Can you work these out from the model? Positions are in its coordinate system, mm. A direction names the side the tool comes from. Round coordinates to 2 decimals unless told otherwise and drop trailing zeros. Loops run counter-clockwise (first coordinate to the right, second up) from the corner with the lowest first, then second, coordinate; pieces in that order, holes last. Notation, with made-up numbers: M 2.25,49 L 13.25,49 A25 cw 13.25,70 Z; hole C 6.25,16 d6. An arc over 180 degrees is marked long. Answer as CSV lines item,"result".
from build123d import *

# Parameters (mm, degrees)
SKETCH1_R           = 26
BOSS_EXTRUDE1_DEPTH = 15
SKETCH3_R           = 15
BOSS_EXTRUDE2_DEPTH = 10
SKETCH4_R           = 11.5
BOSS_EXTRUDE3_DEPTH = 23
SKETCH5_W           = 28
SKETCH5_H           = 12
BOSS_EXTRUDE4_DEPTH = 18
SKETCH6_R           = 1.75
BOSS_EXTRUDE5_DEPTH = 4


with BuildPart() as part:
    # Sketch1 → Boss-Extrude1 (new body)
    with BuildSketch(Plane.XY):
        Circle(SKETCH1_R)
    extrude(amount=BOSS_EXTRUDE1_DEPTH)

    # Sketch2 → Revolve1 (revolve)
    with BuildSketch(Plane(origin=(0, 0, 0), x_dir=(1, 0, 0), z_dir=(0, 1, 0))):
        Polygon((26, -15), (36, -15), (30, -5), (26, -5), align=None)
    revolve(axis=Axis((0, 0, 15), (0, 0, -1)))

    # Sketch3 → Boss-Extrude2 (add)
    with BuildSketch(Plane.XY.offset(15)):
        Circle(SKETCH3_R)
    extrude(amount=BOSS_EXTRUDE2_DEPTH)

    # Sketch4 → Boss-Extrude3 (add)
    with BuildSketch(Plane.XY.offset(25)):
        Circle(SKETCH4_R)
    extrude(amount=BOSS_EXTRUDE3_DEPTH)

    # Sketch5 → Boss-Extrude4 (add)
    with BuildSketch(Plane.XY.offset(48)):
        Rectangle(SKETCH5_W, SKETCH5_H)
    extrude(amount=BOSS_EXTRUDE4_DEPTH)

    # Sketch6 → Boss-Extrude5 (add)
    with BuildSketch(Plane.XY.offset(15)):
        with Locations((-18.75, 0)):
            Circle(SKETCH6_R)
        with Locations(Location((18.75, 0, 0), (0, 0, 180))):
            Circle(SKETCH6_R)
    extrude(amount=BOSS_EXTRUDE5_DEPTH)


solid = part.part
Item 1: If we section it at B-B on x = 0: Write out the boundary of the cut face in (y, z), then the cut area to 4 significant figures.
Output:
outline,"M -36,15 L -30,5 L -26,5 L -26,0 L 26,0 L 26,5 L 30,5 L 36,15 L 15,15 L 15,25 L 11.5,25 L 11.5,48 L 6,48 L 6,66 L -6,66 L -6,48 L -11.5,48 L -11.5,25 L -15,25 L -15,15 Z"
area,"1,965 mm2"
Item 2: We'd pull the mould along Z, two halves only. Please class faces 1 (the face through (0, 0, 0)), 2 (the face through (0, 0, 66)), 3 (the face through (-20.633, -15.821, 2.465)), 4 (the face through (8, -9, 25)): released by +Z, released by -Z, zero draft, split by the parting line, or undercut.
Output:
face 1,"released by -Z"
face 2,"released by +Z"
face 3,"zero draft"
face 4,"undercut"
Item 3: If I drill on line 1 along Z through (x, y) = (0, -11); line 2 along Y through (x, z) = (-8, 55.5); line 3 along Z through (x, y) = (-8, 23), over which ranges is the centre line in solid material (lowest first)? Write a range as from..to.
Output:
line 1,"z = 0..48"
line 2,"y = -6..6"
line 3,"z = 0..15"
Item 4: If we section it at D-D on z = 49: Write out the boundary of the cut face in (x, y), then the cut area to 3 significant figures.
Output:
outline,"M -14,-6 L 14,-6 L 14,6 L -14,6 Z"
area,"336 mm2"
Item 5: If we section it at A-A on y = 0: Write out the boundary of the cut face in (x, z).
Output:
outline,"M -36,15 L -30,5 L -26,5 L -26,0 L 26,0 L 26,5 L 30,5 L 36,15 L 20.5,15 L 20.5,19 L 17,19 L 17,15 L 15,15 L 15,25 L 11.5,25 L 11.5,48 L 14,48 L 14,66 L -14,66 L -14,48 L -11.5,48 L -11.5,25 L -15,25 L -15,15 L -17,15 L -17,19 L -20.5,19 L -20.5,15 Z"
Item 6: On a 3-axis mill with a long thin cutter (end or side, diameter ignored), from which of +Z, -Z, +X, -X, +Y, -Y can I reach the whole of each face in a straight line? I mean faces 5 (the face through (-1.5, 11.4, 36.3)), 6 (the face through (14, 0, 57)), 7 (the face through (-19, 0, 19)), 8 (the face through (0, -8, 48)). Say none if no direction works.
Output:
face 5,"none"
face 6,"+Z, +X, +Y, -Y"
face 7,"+Z, -X, +Y, -Y"
face 8,"+Z, +X, -X, -Y"
Item 7: If we section it at C-C on z = 33: Write out the boundary of the cut face in (x, y).
Output:
outline,"C 0,0 d23"
Item 8: Will these pins go through, and if not, where does the flat tip stop? pin 1 (3 mm diameter, centred on y = 22.5, z = 9.5, fed in from +X); pin 2 (20 mm diameter, centred on x = -2, z = 61, fed in from -Y); pin 3 (8 mm diameter, centred on x = 20.5, y = -15, fed in from +Z).
Output:
pin 1,"stops at x = 25.53"
pin 2,"stops at y = -6"
pin 3,"stops at z = 15"
